Verification items for the finished model (mm, model axes). Coordinates: 2 decimals unless noted, no trailing zeros. Order: outer loops, then holes, each group sorted by start corner. A loop starts at its lowest first (then second) coordinate and runs counter-clockwise, first axis right, second up. Notation, with made-up numbers: (88.25, 37.5) -> (146.25, 37.5) arc R15 ccw to (146.25, 63.5) -> close; hole circle Ø2 at (34, -9.75). An arc over 180 degrees is marked (long way). Use CSV: the item, a comma, the result in double quotes. Start each with the question number.
1) Scan lines: line 1 along X through (y, z) = (34.5, -167); line 2 along Y through (x, z) = (-569, 766); line 3 along Z through (x, y) = (-421, 12.5). Record each from-to range of solid material in increasing order.
2) Go/stop test with flat-tipped pins: pin 1 (12 mm diameter, centred on y = 32, z = 325, fed in from -X); pin 2 (2.5 mm diameter, centred on x = 204, y = 17, fed in from +Z); pin 3 (1.5 mm diameter, centred on x = 210, y = 13.5, fed in from +Z). Record where each tip stops, or that it passes through.
3) Sectioned sample at D-D on y = 31. Record the boundary of the cut face in (x, z).
4) Sectioned sample at B-B on z = -261. Record the boundary of the cut face in (x, y).
5) Sectioned sample at C-C on z = -704. Record the boundary of the cut face in (x, y).
6) Sectioned sample at A-A on x = -263. Record the boundary of the cut face in (y, z), then the cut area to 3 significant figures.
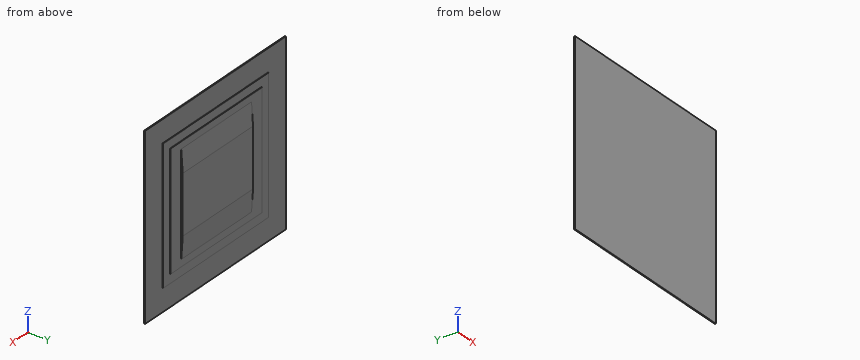
from build123d import *

# Parameters (mm, degrees)
ESQUISSE1_W        = 2000
ESQUISSE1_H        = 2000
BOSS_EXTRU_1_DEPTH = 10
ESQUISSE3_W        = 1500
ESQUISSE3_H        = 1500
BOSS_EXTRU_2_DEPTH = 5
ESQUISSE4_W        = 1300
ESQUISSE4_H        = 1300
BOSS_EXTRU_3_DEPTH = 5
BOSS_EXTRU_5_DEPTH = 500


with BuildPart() as part:
    # Esquisse1 → Boss.-Extru.1 (new body)
    with BuildSketch(Plane(origin=(0, 0, 0), x_dir=(1, 0, 0), z_dir=(0, 1, 0))):
        Rectangle(ESQUISSE1_W, ESQUISSE1_H)
    extrude(amount=BOSS_EXTRU_1_DEPTH)

    # Esquisse3 → Boss.-Extru.2 (add)
    with BuildSketch(Plane(origin=(0, 10, 0), x_dir=(1, 0, 0), z_dir=(0, 1, 0))):
        Rectangle(ESQUISSE3_W, ESQUISSE3_H)
    extrude(amount=BOSS_EXTRU_2_DEPTH)

    # Esquisse4 → Boss.-Extru.3 (add)
    with BuildSketch(Plane(origin=(0, 15, 0), x_dir=(1, 0, 0), z_dir=(0, 1, 0))):
        Rectangle(ESQUISSE4_W, ESQUISSE4_H)
    extrude(amount=BOSS_EXTRU_3_DEPTH)

    # Esquisse8 → Boss.-Extru.5 (add, symmetric)
    with BuildSketch(Plane(origin=(0, 0, 0), x_dir=(0, 0, -1), z_dir=(1, 0, 0))):
        Polygon((325.45099137, 37.196428785), (-325.45099137, 37.196428785), (-571.371380234, 20), (571.371380234, 20), align=None)
    extrude(amount=BOSS_EXTRU_5_DEPTH, both=True)


solid = part.part
Answers follow:
1,line 1,"x = -500 to 500"
1,line 2,"y = 0 to 10"
1,line 3,"z = -750 to 750"
2,pin 1,"stops at x = -500"
2,pin 2,"stops at z = 650"
2,pin 3,"stops at z = 750"
3,outline,"(-500, -414.06) -> (500, -414.06) -> (500, 414.06) -> (-500, 414.06) -> close"
4,outline,"(-1000, 0) -> (1000, 0) -> (1000, 10) -> (750, 10) -> (750, 15) -> (650, 15) -> (650, 20) -> (500, 20) -> (500, 37.2) -> (-500, 37.2) -> (-500, 20) -> (-650, 20) -> (-650, 15) -> (-750, 15) -> (-750, 10) -> (-1000, 10) -> close"
5,outline,"(-1000, 0) -> (1000, 0) -> (1000, 10) -> (750, 10) -> (750, 15) -> (-750, 15) -> (-750, 10) -> (-1000, 10) -> close"
6,outline,"(0, -1000) -> (10, -1000) -> (10, -750) -> (15, -750) -> (15, -650) -> (20, -650) -> (20, -571.37) -> (37.2, -325.45) -> (37.2, 325.45) -> (20, 571.37) -> (20, 650) -> (15, 650) -> (15, 750) -> (10, 750) -> (10, 1000) -> (0, 1000) -> close"
6,area,"49,400 mm²"
